The listing builds one solid part. Answer for the finished solid, in the listing's coordinates (mm). A direction names the side the tool comes from. Give positions to 0.01 mm unless a question says otherwise; leave off trailing zeros. Order: outer loops, then holes, each group sorted by start corner. A loop starts at its lowest first (then second) coordinate and runs counter-clockwise, first axis right, second up. Notation, with made-up numbers: (5.5, -19.75) - (60.5, -19.75) arc R14 ccw to (60.5, -6.75) - close; hole circle Ø2 at (80, 7.5). An arc over 180 degrees is marked (long way). Use a Markdown table: item, result. Add a question column.
1) Find section B-B, the plane z = -13.5. Determine the outline of the cut face in (x, y), plus the area to 3 significant figures.
2) Straight lines are drawn through the part: line 1 (X direction, y = 6.5, z = -21); line 2 (Z direction, x = -3, y = 21); line 3 (Z direction, x = -36.5, y = 11). For each, find the intervals that lie inside material, in ascending order.
3) The mould has two halves that part along X. Classify faces 1 (the face through (-40.2, 14.8, 27.3)), 2 (the face through (36, 9, -13)), 3 (the face through (40.3, 14.8, 27.2)): released by +X, released by -X, zero draft, split by the parting line, or undercut.
4) For faces 4 (the face through (-39, 13, 12)), 5 (the face through (-1, 0, 0)), determine the directions among +Z, -Z, +X, -X, +Y, -Y from which every point of the face is accessible in a straight line to the end or side of a thin tool.
5) Flat-ended cylindrical pins translate along their axes: pin 1 (5.5 mm diameter, centred on x = -39.5, y = 14, fed in from -Z); pin 2 (1.5 mm diameter, centred on x = -2, z = 21, fed in from +Y); pin 3 (4 mm diameter, centred on y = 10.5, z = 26.5, fed in from -X). Find the tip coordinate at first contact, or state that the pin passes through.
6) Find section D-D, the plane x = -18. Determine the outline of the cut face in (y, z), plus the area to 3 significant figures.
7) Find section C-C, the plane x = 32. Determine the outline of the cut face in (y, z), plus the area to 3 significant figures.
8) Find section A-A, the plane y = 3. Determine the outline of the cut face in (x, z), plus the area to 3 significant figures.
from build123d import *

# Parameters (mm, degrees)
SKETCH_3_W                 = 88
SKETCH_3_H                 = 62
EXTRUDE_2_DEPTH            = 30
SHELL_1_T                  = -3
SHELL_1_THICKNESS_2_FACE_W = 56
SHELL_1_THICKNESS_2_FACE_H = 82
SHELL_1_THICKNESS_2_DEPTH  = 2
EXTRUDE_3_DEPTH            = 15
FILLET_1_R                 = 10
CUT_EXTRUDE_1_DEPTH        = 12
EXTRUDE_4_DEPTH            = 20
FILLET_2_R                 = 10
CUT_EXTRUDE_2_DEPTH        = 17
CHAMFER_1_SIZE             = 6
CHAMFER_2_SIZE             = 7.5


with BuildPart() as part:
    # 草图3 → 凸台-拉伸2 (new body)
    with BuildSketch(Plane(origin=(0, 0, 0), x_dir=(1, 0, 0), z_dir=(0, 1, 0))):
        Rectangle(SKETCH_3_W, SKETCH_3_H)
    extrude(amount=EXTRUDE_2_DEPTH)

    # 抽壳1
    shell_1_openings = [part.faces().sort_by_distance(p)[0] for p in [
        (0, 30, 0),
    ]]
    offset(amount=SHELL_1_T, openings=shell_1_openings, kind=Kind.INTERSECTION)

    # 抽壳1 thickness 2 face (on inner face of the shell) → 抽壳1 thickness 2 (add)
    with BuildSketch(Plane(origin=(0, 3, 0), x_dir=(0, 0, -1), z_dir=(0, -1, 0))):
        Rectangle(SHELL_1_THICKNESS_2_FACE_W, SHELL_1_THICKNESS_2_FACE_H)
    extrude(amount=-SHELL_1_THICKNESS_2_DEPTH)

    # 草图5 → 凸台-拉伸3 (add, symmetric)
    with BuildSketch(Plane.XY):
        Polygon((-41, 25), (-41, 5), (-36, 5), (-36, 16.339745962), align=None)
        Polygon((36, 5), (41, 5), (41, 25), (36, 16.339745962), align=None)
    extrude(amount=EXTRUDE_3_DEPTH, both=True)

    # 圆角1
    fillet_1_edges = [part.edges().sort_by_distance(p)[0] for p in [
        (-36, 16.339745962, 0),
        (36, 16.339745962, 0),
    ]]
    fillet(fillet_1_edges, radius=FILLET_1_R)

    # 草图6 → 切除-拉伸1 (cut, symmetric)
    with BuildSketch(Plane.XY):
        Polygon((36, 5), (41, 5), (41, 25), (36, 16.339745962), align=None)
        Polygon((-41, 25), (-41, 5), (-36, 5), (-36, 16.339745962), align=None)
    extrude(amount=CUT_EXTRUDE_1_DEPTH, both=True, mode=Mode.SUBTRACT)

    # 草图7 → 凸台-拉伸4 (add, symmetric)
    with BuildSketch(Plane(origin=(0, 0, 0), x_dir=(0, 0, -1), z_dir=(1, 0, 0))):
        Polygon((-28, 25), (-23, 16.339745962), (-23, 5), (-28, 5), align=None)
        Polygon((23, 5), (28, 5), (28, 25), (23, 16.339745962), align=None)
    extrude(amount=EXTRUDE_4_DEPTH, both=True)

    # 圆角2
    fillet_2_edges = [part.edges().sort_by_distance(p)[0] for p in [
        (0, 16.339745962, 23),
        (0, 16.339745962, -23),
    ]]
    fillet(fillet_2_edges, radius=FILLET_2_R)

    # 草图8 → 切除-拉伸2 (cut, symmetric)
    with BuildSketch(Plane(origin=(0, 0, 0), x_dir=(0, 0, -1), z_dir=(1, 0, 0))):
        Polygon((23, 5), (28, 5), (28, 25), (23, 16.339745962), align=None)
        Polygon((-23, 16.339745962), (-28, 25), (-28, 5), (-23, 5), align=None)
    extrude(amount=CUT_EXTRUDE_2_DEPTH, both=True, mode=Mode.SUBTRACT)

    # 倒角1
    chamfer_1_edges = [part.edges().sort_by_distance(p)[0] for p in [
        (-41, 17.5, -28),
        (-41, 17.5, 28),
        (41, 17.5, 28),
        (41, 17.5, -28),
    ]]
    chamfer(chamfer_1_edges, length=CHAMFER_1_SIZE)

    # 倒角2
    chamfer_2_edges = [part.edges().sort_by_distance(p)[0] for p in [
        (-44, 15, -31),
        (44, 15, -31),
        (44, 15, 31),
        (-44, 15, 31),
    ]]
    chamfer(chamfer_2_edges, length=CHAMFER_2_SIZE)


solid = part.part
The answers:
| question | item | result |
|---|---|---|
| 1 | outline | (-44, 0) - (44, 0) - (44, 30) - (41, 30) - (41, 25) - (37.34, 18.66) arc R10 ccw to (36, 13.66) - (36, 5) - (-36, 5) - (-36, 13.66) arc R10 ccw to (-37.34, 18.66) - (-41, 25) - (-41, 30) - (-44, 30) - close |
| 1 | area | 745 mm2 |
| 2 | line 1 | -44 to -41, 41 to 44 |
| 2 | line 2 | -31 to -28, 28 to 31 |
| 2 | line 3 | -31 to -26.5, -15 to -12, 12 to 15, 26.5 to 31 |
| 3 | face 1 | released by -X |
| 3 | face 2 | undercut |
| 3 | face 3 | released by +X |
| 4 | face 4 | +Y |
| 4 | face 5 | +Z, -Z, +X, -X, -Y |
| 5 | pin 1 | z = -30.75 |
| 5 | pin 2 | y = 5 |
| 5 | pin 3 | x = -43 |
| 6 | outline | (0, -31) - (30, -31) - (30, -28) - (25, -28) - (18.66, -24.34) arc R10 ccw to (13.66, -23) - (5, -23) - (5, 23) - (13.66, 23) arc R10 ccw to (18.66, 24.34) - (25, 28) - (30, 28) - (30, 31) - (0, 31) - close |
| 6 | area | 615 mm2 |
| 7 | outline | (0, -31) - (30, -31) - (30, -28) - (5, -28) - (5, 28) - (30, 28) - (30, 31) - (0, 31) - close |
| 7 | area | 460 mm2 |
| 8 | outline | (-44, -23.5) - (-36.5, -31) - (36.5, -31) - (44, -23.5) - (44, 23.5) - (36.5, 31) - (-36.5, 31) - (-44, 23.5) - close |
| 8 | area | 5,340 mm2 |
